Geometry: final body of the model. Coordinates: model frame, mm. Face numbers are marked on the shaded views. Coordinates: 2 decimals unless noted, no trailing zeros. Loops run counter-clockwise (first coordinate to the right, second up) from the corner with the lowest first, then second, coordinate; pieces in that order, holes last. Notation, with made-up numbers: (59.25, 64) - (113.25, 64) arc R30 cw to (113.25, 92) - close; hole circle Ø4 at (48.25, -3.75). An arc over 180 degrees is marked (long way). Put each result on its own line as item: value. Start each with the question number.
1) Section B-B on z = 178. Output: boundary loops of the cut face in (x, y).
2) Contact query for flat-ended pins moving along their axis: pin 1 Ø2 at (y, z) = (16, 281) entering from -X; pin 2 Ø1.3 at (y, z) = (-16, 301.5) entering from +X; pin 3 Ø1.9 at (y, z) = (-18, 40.5) entering from -X. Output: stop coordinate, or through.
3) Section A-A on z = 240. Output: boundary loops of the cut face in (x, y).
4) Draft query along Z for the marked faces 1 and 2. Return one class per face: +Z half, -Z half, draft (parallel to the pull), parting line (faces both ways), or undercut.
5) Section C-C on z = 43.5. Output: boundary loops of the cut face in (x, y) (3 decimals).
6) Material intervals for line 1 along Y through (x, z) = (0, 12.5); line 2 along X through (y, z) = (0, 13); line 3 along Z through (x, y) = (22.5, -8), sorted ascending. Write a range as from..to.
```python
from build123d import *
from build123d.topology import SkipClean

# Parameters (mm, degrees)
SKICA1_R                  = 20
P_IDAT_VYSUNUT_M1_DEPTH   = 66
SKICA2_R                  = 27.5
P_IDAT_VYSUNUT_M2_DEPTH   = 35
SKICA3_R                  = 26.5
P_IDAT_VYSUNUT_M3_DEPTH   = 84
SKICA4_R                  = 27.5
P_IDAT_VYSUNUT_M4_DEPTH   = 35
SKICA5_R                  = 20
P_IDAT_VYSUNUT_M5_DEPTH   = 30
SKICA6_R                  = 17.5
P_IDAT_VYSUNUT_M6_DEPTH   = 90
ZKOSEN_3_SIZE             = 6
ZKOSEN_3_SIZE2            = 3.464101615
SKICA9_OUTSIDE_W          = 126.756
SKICA9_OUTSIDE_H          = 126.756
ODEBRAT_VYSUNUT_M16_DEPTH = 90
ZKOSEN_4_SIZE             = 0.5
M10_Z_VIT1_D              = 8.5
M10_Z_VIT1_DEPTH          = 30
M10_Z_VIT1_TIP            = 2.553657631
ODEBRAT_START             = -15
ODEBRAT_VYSUNUT_M17_DEPTH = 13.5


with BuildPart() as part:
    # Skica1 → P_idat vysunut_m1 (new body)
    with BuildSketch(Plane.XY):
        Circle(SKICA1_R)
    extrude(amount=P_IDAT_VYSUNUT_M1_DEPTH)

    # Skica2 → P_idat vysunut_m2 (add)
    with BuildSketch(Plane.XY.offset(66)):
        Circle(SKICA2_R)
    extrude(amount=P_IDAT_VYSUNUT_M2_DEPTH)

    # Skica3 → P_idat vysunut_m3 (add)
    with BuildSketch(Plane.XY.offset(101)):
        Circle(SKICA3_R)
    extrude(amount=P_IDAT_VYSUNUT_M3_DEPTH)

    # Skica4 → P_idat vysunut_m4 (add)
    with BuildSketch(Plane.XY.offset(185)):
        Circle(SKICA4_R)
    extrude(amount=P_IDAT_VYSUNUT_M4_DEPTH)

    # Skica5 → P_idat vysunut_m5 (add)
    with BuildSketch(Plane.XY.offset(220)):
        Circle(SKICA5_R)
    extrude(amount=P_IDAT_VYSUNUT_M5_DEPTH)

    # Skica6 → P_idat vysunut_m6 (add)
    with BuildSketch(Plane.XY.offset(250)):
        Circle(SKICA6_R)
    extrude(amount=P_IDAT_VYSUNUT_M6_DEPTH)

    # Zkosen_3
    zkosen_3_edges = [part.edges().sort_by_distance(p)[0] for p in [
        (-17.5, 0, 340),
    ]]
    zkosen_3_side = [part.faces().sort_by_distance(p)[0] for p in [
        (-17.5, 0, 295),
    ]]
    chamfer(zkosen_3_edges, length=ZKOSEN_3_SIZE, length2=ZKOSEN_3_SIZE2, reference=zkosen_3_side[0])

    # Skica9 outside → Odebrat vysunut_m16 (cut)
    with BuildSketch(Plane.XY.offset(340)):
        Rectangle(SKICA9_OUTSIDE_W, SKICA9_OUTSIDE_H)
        with BuildLine():
            Line((-4.25, 14.385322381), (-4.25, 16.976086121))
            ThreePointArc((-4.25, 16.976086121), (0, 17.5), (4.25, 16.976086121))
            Line((4.25, 16.976086121), (4.25, 14.385322381))
            ThreePointArc((4.25, 14.385322381), (7.5, 12.990381057), (10.333054623, 10.873269156))
            Line((10.333054623, 10.873269156), (12.576721838, 12.168651027))
            ThreePointArc((12.576721838, 12.168651027), (15.155444566, 8.75), (16.826721838, 4.807435095))
            Line((16.826721838, 4.807435095), (14.583054623, 3.512053224))
            ThreePointArc((14.583054623, 3.512053224), (15, 0), (14.583054623, -3.512053224))
            Line((14.583054623, -3.512053224), (16.826721838, -4.807435095))
            ThreePointArc((16.826721838, -4.807435095), (15.155444566, -8.75), (12.576721838, -12.168651027))
            Line((12.576721838, -12.168651027), (10.333054623, -10.873269156))
            ThreePointArc((10.333054623, -10.873269156), (7.5, -12.990381057), (4.25, -14.385322381))
            Line((4.25, -14.385322381), (4.25, -16.976086121))
            ThreePointArc((4.25, -16.976086121), (0, -17.5), (-4.25, -16.976086121))
            Line((-4.25, -16.976086121), (-4.25, -14.385322381))
            ThreePointArc((-4.25, -14.385322381), (-7.5, -12.990381057), (-10.333054623, -10.873269156))
            Line((-10.333054623, -10.873269156), (-12.576721838, -12.168651027))
            ThreePointArc((-12.576721838, -12.168651027), (-15.155444566, -8.75), (-16.826721838, -4.807435095))
            Line((-16.826721838, -4.807435095), (-14.583054623, -3.512053224))
            ThreePointArc((-14.583054623, -3.512053224), (-15, 0), (-14.583054623, 3.512053224))
            Line((-14.583054623, 3.512053224), (-16.826721838, 4.807435095))
            ThreePointArc((-16.826721838, 4.807435095), (-15.155444566, 8.75), (-12.576721838, 12.168651027))
            Line((-12.576721838, 12.168651027), (-10.333054623, 10.873269156))
            ThreePointArc((-10.333054623, 10.873269156), (-7.5, 12.990381057), (-4.25, 14.385322381))
        make_face(mode=Mode.SUBTRACT)
    extrude(amount=-ODEBRAT_VYSUNUT_M16_DEPTH, mode=Mode.SUBTRACT)

    # Zkosen_4
    zkosen_4_edges = [part.edges().sort_by_distance(p)[0] for p in [
        (-27.5, 0, 185),
        (-27.5, 0, 220),
        (-20, 0, 0),
        (-20, 0, 250),
        (-27.5, 0, 66),
        (-27.5, 0, 101),
    ]]
    chamfer(zkosen_4_edges, length=ZKOSEN_4_SIZE)

    # M10 z_vit1
    with Locations(Plane(origin=(0, 0, 0), x_dir=(-1, 0, 0), z_dir=(0, 0, -1))):
        with Locations((0, 0)):
            Hole(M10_Z_VIT1_D / 2, depth=M10_Z_VIT1_DEPTH)
            with Locations((0, 0, -(M10_Z_VIT1_DEPTH + M10_Z_VIT1_TIP / 2))):  # 118° drill point
                Cone(0, M10_Z_VIT1_D / 2, M10_Z_VIT1_TIP, mode=Mode.SUBTRACT)

    # Skica12 → Odebrat vysunut_m17 (cut, through all)
    with SkipClean():  # keep this step's faces unmerged: merging them makes the solid invalid here
        with BuildSketch(Plane(origin=(0, 0, 0), x_dir=(1, 0, 0), z_dir=(0, 1, 0)).offset(ODEBRAT_START)):
            with BuildLine():
                Line((-7, 0), (-7, -58.99999898))
                ThreePointArc((-7, -58.99999898), (0, -66), (7, -58.99999898))
                Line((7, -58.99999898), (7, 0))
                Line((7, 0), (-7, 0))
            make_face()
        extrude(amount=-ODEBRAT_VYSUNUT_M17_DEPTH, mode=Mode.SUBTRACT)


solid = part.part
```
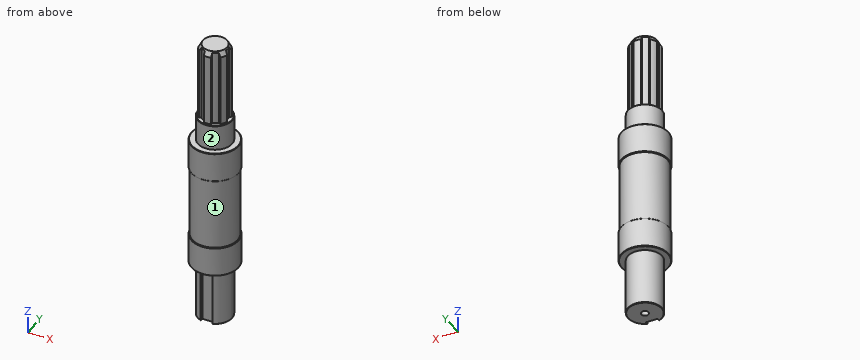
Answer block:
1. outline: circle Ø53 at (0, 0)
2. pin 1: stops at x = -4.25
2. pin 2: stops at x = 4.25
2. pin 3: stops at x = -10.45
3. outline: circle Ø40 at (0, 0)
4. face 1: undercut
4. face 2: draft
5. outline: (-7, -18.735) - (-7, -15) - (7, -15) - (7, -18.735) arc R20 ccw (long way) to start
6. line 1: y = -15..-4.25, 4.25..20
6. line 2: x = -20..-4.25, 4.25..20
6. line 3: z = 66..220
